Could you check a few things on this drawing? It's one solid part, dimensions in mm from its lowest x, y, z. Round coordinates to 2 decimals unless told otherwise and drop trailing zeros. Write each loop counter-clockwise with the first axis right and the second up, starting at its lowest first coordinate (ties: lowest second). Pieces come first, ordered by that corner, then holes. Notation, with made-up numbers: M -16,-33.75 L 5,-33.75 A20 cw 5,-1.75 Z; hole C 13.5,51 d1. An arc over 180 degrees is marked long. One line per question, with ' | ' between items. Start each with the question number.
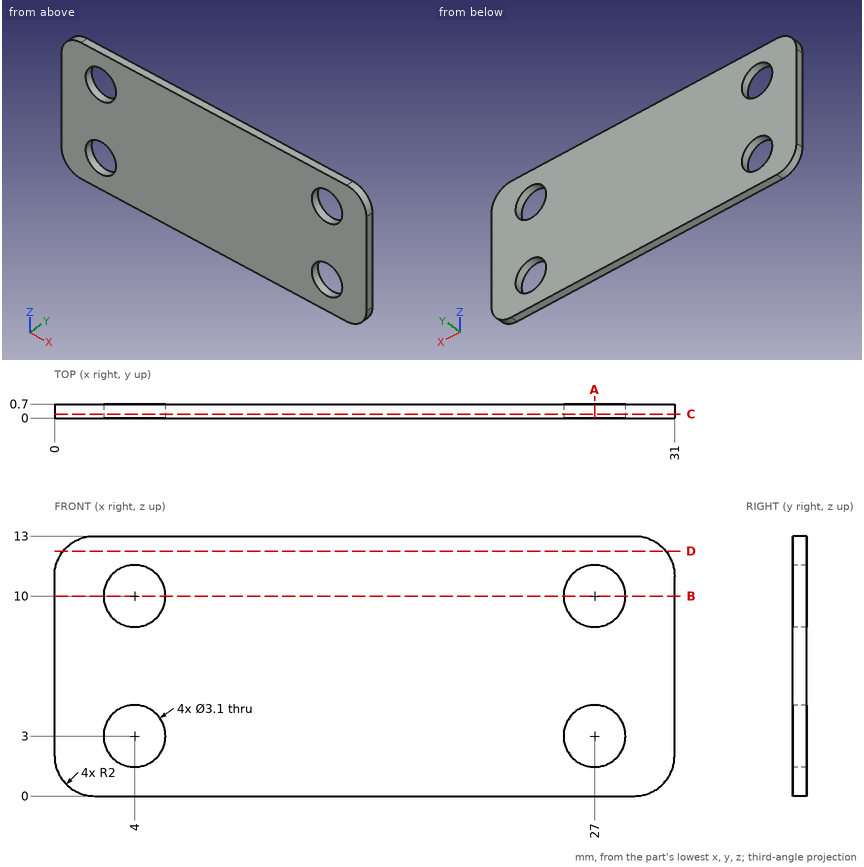
1. Suppose I cut it at A-A (x = 27). Write out the boundary of the cut face in (y, z).
2. Suppose I cut it at B-B (z = 10). Write out the boundary of the cut face in (x, y).
3. I need wall thicknesses on line 1 along Z through (x, y) = (4, 0.35); line 2 along X through (y, z) = (0.1, 12). Which ranges of each line are inside material? Lowest first, please. Write a range as from..to.
4. Suppose I cut it at D-D (z = 12.25). Write out the boundary of the cut face in (x, y), and give its area (3 significant figures).
5. Suppose I cut it at C-C (y = 0.2). Write out the boundary of the cut face in (x, z).
Computed:
1) outline: M 0,0 L 0.7,0 L 0.7,1.45 L 0,1.45 Z; M 0,4.55 L 0.7,4.55 L 0.7,8.45 L 0,8.45 Z; M 0,11.55 L 0.7,11.55 L 0.7,13 L 0,13 Z
2) outline: M 0,0 L 2.45,0 L 2.45,0.7 L 0,0.7 Z; M 5.55,0 L 25.45,0 L 25.45,0.7 L 5.55,0.7 Z; M 28.55,0 L 31,0 L 31,0.7 L 28.55,0.7 Z
3) line 1: z = 0..1.45, 4.55..8.45, 11.55..13 | line 2: x = 0.27..30.73
4) outline: M 0.44,0 L 30.56,0 L 30.56,0.7 L 0.44,0.7 Z | area: 21.1 mm²
5) outline: M 0,2 A2 ccw 2,0 L 29,0 A2 ccw 31,2 L 31,11 A2 ccw 29,13 L 2,13 A2 ccw 0,11 Z; hole C 4,3 d3.1; hole C 4,10 d3.1; hole C 27,3 d3.1; hole C 27,10 d3.1
